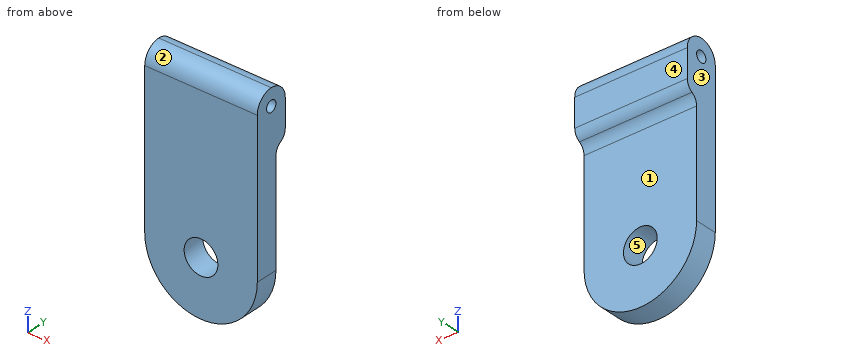
from build123d import *

# Parameters (mm, degrees)
SALIENTE_EXTRUIR1_DEPTH = 3
CROQUIS3_W              = 15
CROQUIS3_H              = 1
CORTAR_EXTRUIR1_DEPTH   = 10
REDONDEO1_R             = 1
REDONDEO3_R             = 1
CROQUIS4_R              = 0.5
CORTAR_EXTRUIR2_DEPTH   = 10
REDONDEO4_R             = 1.5
REDONDEO5_R             = 1.5
CROQUIS5_R              = 1.5
CORTAR_EXTRUIR3_DEPTH   = 3


with BuildPart() as part:
    # Croquis1 → Saliente-Extruir1 (new body)
    with BuildSketch(Plane(origin=(0, 0, 0), x_dir=(1, 0, 0), z_dir=(0, 1, 0))):
        with BuildLine():
            Line((0, 0), (10, 0))
            Line((10, 0), (10, 15))
            ThreePointArc((10, 15), (5, 20), (0, 15))
            Line((0, 15), (0, 0))
        make_face()
    extrude(amount=SALIENTE_EXTRUIR1_DEPTH)

    # Croquis3 → Cortar-Extruir1 (cut)
    with BuildSketch(Plane(origin=(0, 0, 0), x_dir=(0, 0, -1), z_dir=(1, 0, 0))):
        with Locations((12.5, 2.5)):
            Rectangle(CROQUIS3_W, CROQUIS3_H)
    extrude(amount=CORTAR_EXTRUIR1_DEPTH, mode=Mode.SUBTRACT)

    # Redondeo1
    redondeo1_edges = [part.edges().sort_by_distance(p)[0] for p in [
        (5, 3, -5),
    ]]
    fillet(redondeo1_edges, radius=REDONDEO1_R - 0.0001)  # a hair under: the kernel refuses the full size

    # Redondeo3
    redondeo3_edges = [part.edges().sort_by_distance(p)[0] for p in [
        (5, 2, -5),
    ]]
    fillet(redondeo3_edges, radius=REDONDEO3_R)

    # Croquis4 → Cortar-Extruir2 (cut)
    with BuildSketch(Plane(origin=(10, 0, 0), x_dir=(0, 0, -1), z_dir=(1, 0, 0))):
        with Locations((1.5, 1.5)):
            Circle(CROQUIS4_R)
    extrude(amount=-CORTAR_EXTRUIR2_DEPTH, mode=Mode.SUBTRACT)

    # Redondeo4
    redondeo4_edges = [part.edges().sort_by_distance(p)[0] for p in [
        (5, 3, 0),
    ]]
    fillet(redondeo4_edges, radius=REDONDEO4_R)

    # Redondeo5
    redondeo5_edges = [part.edges().sort_by_distance(p)[0] for p in [
        (5, 0, 0),
    ]]
    fillet(redondeo5_edges, radius=REDONDEO5_R - 0.0001)  # a hair under: the kernel refuses the full size

    # Croquis5 → Cortar-Extruir3 (cut)
    with BuildSketch(Plane(origin=(0, 2, 0), x_dir=(1, 0, 0), z_dir=(0, 1, 0))):
        with Locations(Location((5, 15, 0), (0, 0, 270))):
            Circle(CROQUIS5_R)
    extrude(amount=-CORTAR_EXTRUIR3_DEPTH, mode=Mode.SUBTRACT)


solid = part.part
Build history of the part. All positions in model axes, mm. Face numbers are marked on the shaded views. A direction names the side the tool comes from. Coordinates: 2 decimals unless noted, no trailing zeros. Write each loop counter-clockwise with the first axis right and the second up, starting at its lowest first coordinate (ties: lowest second). Pieces come first, ordered by that corner, then holes.
(1) Cut at B-B on z = -7.75. List the corners of the cut face in (x, y).
(2) 3-axis set-ups, long thin cutter, end or side, ignore diameter. For the marked faces 1 and 2: which of +Z, -Z, +X, -X, +Y, -Y reach the whole face in a straight line?
(3) Mould opens along X. For the marked faces 3, 4 and 5 say: pulls with the +X half, pulls with the -X half, needs draft (parallel to the pull), parting line crosses it, or undercut.
(4) Cut at A-A on x = 5. State how many separate pieces and enclosed holes the cut face has, and give its area (3 significant figures).
(5) Pin check, flat tip, straight feed: pin 1 Ø5 at (x, z) = (3.5, -10) entering from +Y. Stop position of the tip, or through.
(6) Drill centre lines: line 1 (X direction, y = 1.05, z = -15); line 2 (Y direction, x = 1.5, z = -7.5); line 3 (Z direction, x = 1.75, y = 1.3). Where is each one in solid material? Low to high.
Working result:
1. outline: (0, 0) - (10, 0) - (10, 2) - (0, 2) - close
2. face 1: -Z, +X, -X, +Y
2. face 2: +Z, +X, -X, -Y
3. face 3: pulls with the -X half
3. face 4: needs draft
3. face 5: undercut
4. separate pieces: 2
4. enclosed holes: 1
4. area: 37.1 mm2
5. pin 1: stops at y = 2
6. line 1: x = 0 to 3.5, 6.5 to 10
6. line 2: y = 0 to 2
6. line 3: z = -18.8 to -1.96, -1.04 to -0.01
